Source: three-view drawing plus pictorial views. Frame: mm from the lowest corner of the part. Give positions to 0.01 mm unless a question says otherwise; leave off trailing zeros. Loops run counter-clockwise (first coordinate to the right, second up) from the corner with the lowest first, then second, coordinate; pieces in that order, holes last. Notation, with made-up numbers: (66.25, 23.5) -> (89.25, 23.5) arc R12 cw to (89.25, 30.5) -> close; hole circle Ø10 at (80.5, -13). An arc over 180 degrees is marked (long way). One line per item, written item: value. Start each with the question number.
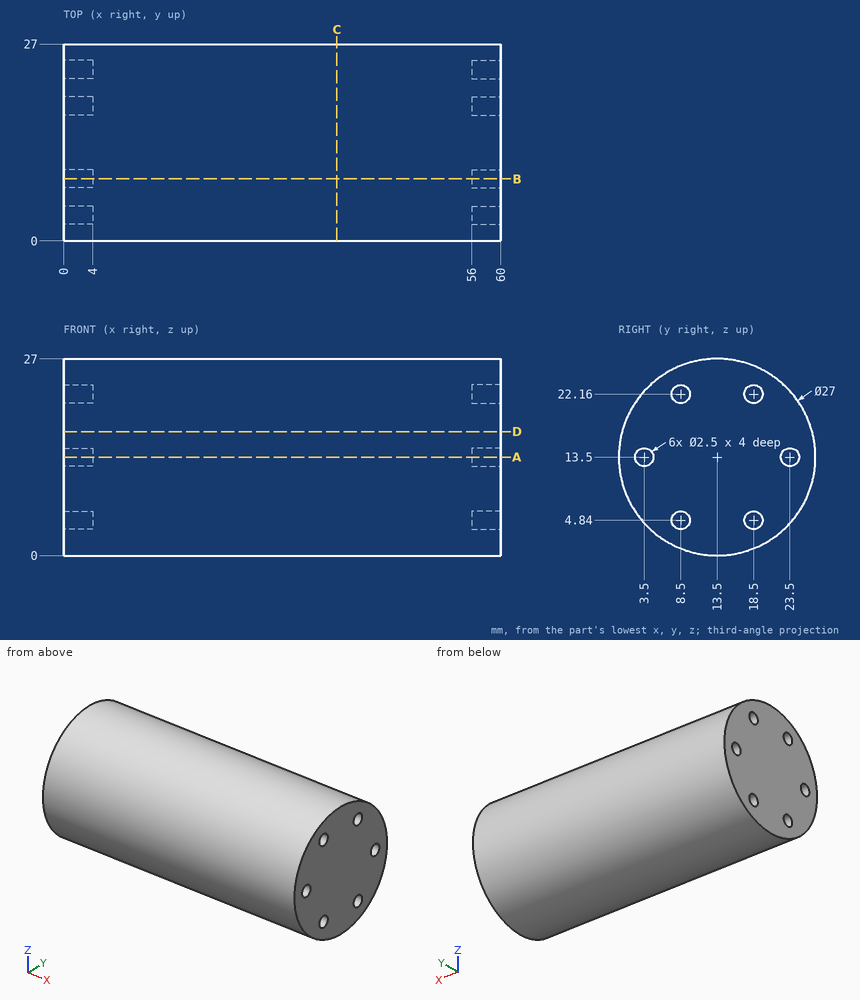
Item 1: Pin query (flat end, axial travel): pin 1 (2 mm diameter, centred on y = 3.5, z = 13, fed in from +X); pin 2 (2 mm diameter, centred on y = 18.5, z = 4.84, fed in from -X); pin 3 (1.5 mm diameter, centred on x = 23, y = 22, fed in from -Z); pin 4 (6 mm diameter, centred on x = 45, z = 18.5, fed in from -Y). Return the tip coordinate at first contact, or that it passes through.
Item 2: Section C-C, the plane x = 37.5. Output: boundary loops of the cut face in (y, z).
Item 3: Section A-A, the plane z = 13.5. Output: boundary loops of the cut face in (x, y), then the cut area to 3 significant figures.
Item 4: Section D-D, the plane z = 17. Output: boundary loops of the cut face in (x, y), then the cut area to 3 significant figures.
Item 5: Ray query, line 1 along Y through (x, z) = (1.5, 13.5); line 2 along Z through (x, y) = (2.5, 19.5) (1 decimal); line 3 along X through (y, z) = (24.5, 13). Return the intervals inside material, ascending. Write a range as [from, to].
Item 6: Section B-B, the plane y = 8.5. Output: boundary loops of the cut face in (x, z), then the cut area to 3 significant figures.
Geometry check:
1. pin 1: stops at x = 60
1. pin 2: stops at x = 4
1. pin 3: stops at z = 2.45
1. pin 4: stops at y = 0.15
2. outline: circle Ø27 at (13.5, 13.5)
3. outline: (0, 0) -> (60, 0) -> (60, 2.25) -> (56, 2.25) -> (56, 4.75) -> (60, 4.75) -> (60, 22.25) -> (56, 22.25) -> (56, 24.75) -> (60, 24.75) -> (60, 27) -> (0, 27) -> (0, 24.75) -> (4, 24.75) -> (4, 22.25) -> (0, 22.25) -> (0, 4.75) -> (4, 4.75) -> (4, 2.25) -> (0, 2.25) -> close
3. area: 1,580 mm2
4. outline: (0, 0.46) -> (60, 0.46) -> (60, 26.54) -> (0, 26.54) -> close
4. area: 1,560 mm2
5. line 1: y = [0, 2.25], [4.75, 22.25], [24.75, 27]
5. line 2: z = [1.4, 4.1], [5.6, 21.4], [22.9, 25.6]
5. line 3: x = [4, 56]
6. outline: (0, 0.96) -> (60, 0.96) -> (60, 3.59) -> (56, 3.59) -> (56, 6.09) -> (60, 6.09) -> (60, 20.91) -> (56, 20.91) -> (56, 23.41) -> (60, 23.41) -> (60, 26.04) -> (0, 26.04) -> (0, 23.41) -> (4, 23.41) -> (4, 20.91) -> (0, 20.91) -> (0, 6.09) -> (4, 6.09) -> (4, 3.59) -> (0, 3.59) -> close
6. area: 1,460 mm2
